Check sheet for the modelled part. Datum: model origin and axes. Units: mm. Face numbers are marked on the shaded views. A direction names the side the tool comes from. Give positions to 0.01 mm unless a question says otherwise; leave off trailing zeros. Order: outer loops, then holes, each group sorted by start corner. A loop starts at its lowest first (then second) coordinate and runs counter-clockwise, first axis right, second up. Notation, with made-up numbers: (21.25, 43.25) -> (69.25, 43.25) arc R13 cw to (69.25, 60.25) -> close; hole circle Ø1 at (45, 89.25). An arc over 180 degrees is marked (long way). Answer in a Markdown table with one row per item. Add a question column.
(1) Cross-section at B-B (x = 0). Record the cut outline in (y, z), then the cut area to 3 significant figures.
(2) Go/stop test with flat-tipped pins: pin 1 (8 mm diameter, centred on y = 6.5, z = 4.5, fed in from +X); pin 2 (1 mm diameter, centred on x = 15, z = 6, fed in from -Y); pin 3 (8.5 mm diameter, centred on x = 0, y = 23.75, fed in from +Z); pin 4 (12 mm diameter, centred on x = -6, y = 20, fed in from -Z). Record where each tip stops, or that it passes through.
(3) Set-up check for the marked faces 4 and 5: record each of +Z, -Z, +X, -X, +Y, -Y from which the full face is reachable in a straight line by a thin tool's end or side.
(4) Cross-section at C-C (z = 10.5). Record the cut outline in (x, y).
(5) Thickness scan on L1, parallel to Y at x = 0, z = 3.05; L2, parallel to X at y = -11, z = 3.75; L3, parallel to Z at x = -27, y = -2.5. Record the ranges inside material, lowest first. Write a range as [from, to].
(6) Cross-section at D-D (y = 7.5). Record the cut outline in (x, z), then the cut area to 3 significant figures.
(7) Release check for a two-part mould opening along Y. For the marked faces 1, 2 and 3 record: released by +Y, released by -Y, zero draft, split by the parting line, or undercut.
(8) Cross-section at A-A (y = 0). Record the cut outline in (x, z).
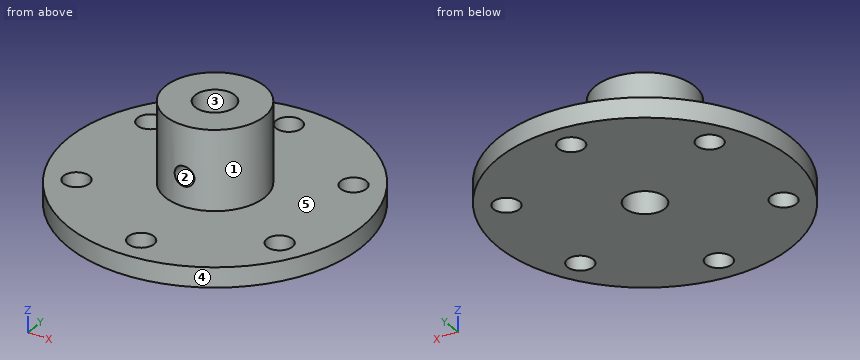
```python
from build123d import *

# Parameters (mm, degrees)
SKETCH1_R               = 29.5
BOSS_EXTRUDE1_DEPTH     = 4
SKETCH2_R               = 10
BOSS_EXTRUDE2_DEPTH     = 16
SKETCH3_R               = 4
CUT_EXTRUDE1_DEPTH      = 20
SKETCH4_R               = 2.6
CUT_EXTRUDE2_DEPTH      = 4
CUT_EXTRUDE3_DEPTH      = 47.265537931
CUT_EXTRUDE3_DEPTH_BACK = 47.265537931
SKETCH5_R               = 2


with BuildPart() as part:
    # Sketch1 → Boss-Extrude1 (new body)
    with BuildSketch(Plane.XY):
        Circle(SKETCH1_R)
    extrude(amount=BOSS_EXTRUDE1_DEPTH)

    # Sketch2 → Boss-Extrude2 (add)
    with BuildSketch(Plane.XY.offset(4)):
        Circle(SKETCH2_R)
    extrude(amount=BOSS_EXTRUDE2_DEPTH)

    # Sketch3 → Cut-Extrude1 (cut)
    with BuildSketch(Plane.XY.offset(20)):
        Circle(SKETCH3_R)
    extrude(amount=-CUT_EXTRUDE1_DEPTH, mode=Mode.SUBTRACT)

    # Sketch4 → Cut-Extrude2 (cut)
    with BuildSketch(Plane.XY.offset(4)):
        with Locations((0, 23.75)):
            Circle(SKETCH4_R)
        with Locations((20.56810334, 11.875)):
            Circle(SKETCH4_R)
        with Locations((20.56810334, -11.875)):
            Circle(SKETCH4_R)
        with Locations((0, -23.75)):
            Circle(SKETCH4_R)
        with Locations((-20.56810334, -11.875)):
            Circle(SKETCH4_R)
        with Locations((-20.56810334, 11.875)):
            Circle(SKETCH4_R)
    extrude(amount=-CUT_EXTRUDE2_DEPTH, mode=Mode.SUBTRACT)

    # Sketch5 → Cut-Extrude3 (cut, two sides: drawn at the far end of the back side and taken through both)
    with BuildSketch(Plane(origin=(0, 0, 0), x_dir=(1, 0, 0), z_dir=(0, 1, 0)).offset(-CUT_EXTRUDE3_DEPTH_BACK)):
        with Locations(Location((0, -10, 0), (0, 0, 270))):
            Circle(SKETCH5_R)
    extrude(amount=CUT_EXTRUDE3_DEPTH + CUT_EXTRUDE3_DEPTH_BACK, mode=Mode.SUBTRACT)


solid = part.part
```
Answer below:
| question | item | result |
|---|---|---|
| 1 | outline | (-29.5, 0) -> (-26.35, 0) -> (-26.35, 4) -> (-29.5, 4) -> close; (-21.15, 0) -> (-4, 0) -> (-4, 8) -> (-10, 8) -> (-10, 4) -> (-21.15, 4) -> close; (-10, 12) -> (-4, 12) -> (-4, 20) -> (-10, 20) -> close; (4, 0) -> (21.15, 0) -> (21.15, 4) -> (10, 4) -> (10, 8) -> (4, 8) -> close; (4, 12) -> (10, 12) -> (10, 20) -> (4, 20) -> close; (26.35, 0) -> (29.5, 0) -> (29.5, 4) -> (26.35, 4) -> close |
| 1 | area | 306 mm² |
| 2 | pin 1 | stops at x = 29.39 |
| 2 | pin 2 | passes through |
| 2 | pin 3 | stops at z = 4 |
| 2 | pin 4 | stops at z = 0 |
| 3 | face 4 | +Z, -Z |
| 3 | face 5 | +Z |
| 4 | outline | (-1.94, -9.81) -> (-1.94, -3.5) arc R4 cw to (-1.94, 3.5) -> (-1.94, 9.81) arc R10 ccw to start; (1.94, -9.81) arc R10 ccw to (1.94, 9.81) -> (1.94, 3.5) arc R4 cw to (1.94, -3.5) -> close |
| 5 | L1 | y = [-29.5, -26.35], [-21.15, -4], [4, 21.15], [26.35, 29.5] |
| 5 | L2 | x = [-27.37, -23.02], [-18.12, 18.12], [23.02, 27.37] |
| 5 | L3 | z = [0, 4] |
| 6 | outline | (-28.53, 0) -> (28.53, 0) -> (28.53, 4) -> (6.61, 4) -> (6.61, 20) -> (-6.61, 20) -> (-6.61, 4) -> (-28.53, 4) -> close; hole circle Ø4 at (0, 10) |
| 6 | area | 427 mm² |
| 7 | face 1 | split by the parting line |
| 7 | face 2 | zero draft |
| 7 | face 3 | undercut |
| 8 | outline | (-29.5, 0) -> (-4, 0) -> (-4, 20) -> (-10, 20) -> (-10, 4) -> (-29.5, 4) -> close; (4, 0) -> (29.5, 0) -> (29.5, 4) -> (10, 4) -> (10, 20) -> (4, 20) -> close |
